Work out the finished part from the listing and answer in its coordinate system (mm). Give positions to 0.01 mm unless a question says otherwise; leave off trailing zeros. Loops run counter-clockwise (first coordinate to the right, second up) from the corner with the lowest first, then second, coordinate; pieces in that order, holes last. Notation, with made-up numbers: (89.25, -34.5) - (134.25, -34.5) arc R22 cw to (134.25, -11.5) - close; hole circle Ø6 at (67.25, 35). An arc over 180 degrees is marked (long way). One line per item, written item: value.
from build123d import *

# Parameters (mm, degrees)
SKETCH1_R           = 1.599999998
SKETCH1_R_2         = 1.45
BOSS_EXTRUDE1_DEPTH = 2


with BuildPart() as part:
    # Sketch1 → Boss-Extrude1 (new body)
    with BuildSketch(Plane.XZ):
        with BuildLine():
            Line((16.181421483, -3.177760966), (9.872858324, -4.530534353))
            ThreePointArc((9.872858324, -4.530534353), (9.325880949, -4.494155653), (8.88026758, -4.174880875))
            ThreePointArc((8.88026758, -4.174880875), (8.049335418, -3.798153126), (7.258365077, -4.252837604))
            ThreePointArc((7.258365077, -4.252837604), (6.336866412, -4.705264718), (5.502330147, -4.107435892))
            ThreePointArc((5.502330147, -4.107435892), (0, -0.499999997), (-5.502330147, -4.107435892))
            ThreePointArc((-5.502330147, -4.107435892), (-6.336866412, -4.705264718), (-7.258365077, -4.252837604))
            ThreePointArc((-7.258365077, -4.252837604), (-8.049335418, -3.798153126), (-8.88026758, -4.174880875))
            ThreePointArc((-8.88026758, -4.174880875), (-9.325880949, -4.494155653), (-9.872858324, -4.530534353))
            Line((-9.872858324, -4.530534353), (-16.181421483, -3.177760966))
            ThreePointArc((-16.181421483, -3.177760966), (-18.749999999, 0), (-16.181421483, 3.177760966))
            Line((-16.181421483, 3.177760966), (-7.150681086, 5.114262981))
            ThreePointArc((-7.150681086, 5.114262981), (-6.698238018, 5.106573021), (-6.295506482, 4.900245189))
            ThreePointArc((-6.295506482, 4.900245189), (-5.464959808, 4.681269053), (-4.770928095, 5.187310858))
            ThreePointArc((-4.770928095, 5.187310858), (-4.48101085, 5.518641983), (-4.076896383, 5.693352662))
            Line((-4.076896383, 5.693352662), (-1.17489874, 6.239775137))
            ThreePointArc((-1.17489874, 6.239775137), (0, 6.34942366), (1.17489874, 6.239775137))
            Line((1.17489874, 6.239775137), (4.076896383, 5.693352662))
            ThreePointArc((4.076896383, 5.693352662), (4.48101085, 5.518641983), (4.770928095, 5.187310858))
            ThreePointArc((4.770928095, 5.187310858), (5.464959808, 4.681269053), (6.295506482, 4.900245189))
            ThreePointArc((6.295506482, 4.900245189), (6.698238018, 5.106573021), (7.150681086, 5.114262981))
            Line((7.150681086, 5.114262981), (16.181421483, 3.177760966))
            ThreePointArc((16.181421483, 3.177760966), (18.749999999, 0), (16.181421483, -3.177760966))
        make_face()
        with Locations(Location((-15.5, 0, 0), (0, 0, 90))):
            Circle(SKETCH1_R, mode=Mode.SUBTRACT)
        with Locations(Location((15.5, 0, 0), (0, 0, 270))):
            Circle(SKETCH1_R, mode=Mode.SUBTRACT)
        with Locations(Location((7.931558887, -1.04420954, 0), (0, 0, 270))):
            Circle(SKETCH1_R_2, mode=Mode.SUBTRACT)
        with Locations(Location((-7.931558887, -1.04420954, 0), (0, 0, 90))):
            Circle(SKETCH1_R_2, mode=Mode.SUBTRACT)
    extrude(amount=-BOSS_EXTRUDE1_DEPTH)


solid = part.part
1. A flat-ended cylindrical pin translates along its axis: pin 1 Ø1 at (x, y) = (8, 0.5) entering from -Z (3 decimals). Find the tip coordinate at first contact, or state that the pin passes through.
Output:
pin 1: stops at z = -3.995
2. Section A-A (z = -1.25) is taken. Write down the section's boundary in (x, y).
Output:
outline: (-18.5, 0) - (-16.5, 0) - (-16.5, 2) - (-18.5, 2) - close; (-14.5, 0) - (-9.37, 0) - (-9.37, 2) - (-14.5, 2) - close; (-6.5, 0) - (-2.9, 0) - (-2.9, 2) - (-6.5, 2) - close; (2.9, 0) - (6.5, 0) - (6.5, 2) - (2.9, 2) - close; (9.37, 0) - (14.5, 0) - (14.5, 2) - (9.37, 2) - close; (16.5, 0) - (18.5, 0) - (18.5, 2) - (16.5, 2) - close
3. Find the intervals of material crossed by line 1 along X through (y, z) = (1.5, 0); line 2 along X through (y, z) = (0.45, -2); line 3 along X through (y, z) = (1.7, 1.25), in increasing order.
Output:
line 1: x = -18.75 to -17.1, -13.9 to -8.94, -6.93 to 6.93, 8.94 to 13.9, 17.1 to 18.75
line 2: x = -18.06 to -9.02, -6.84 to -3.97, 3.97 to 6.84, 9.02 to 18.06
line 3: x = -18.5 to -16.5, -14.5 to 14.5, 16.5 to 18.5
4. The mould has two halves that part along Z. Classify faces 1 (the cylindrical face through (17.086, 0.986, 0.208)), 2 (the cylindrical face through (0.1, 1, -0.5)), 3 (the flat face through (11.6, 0.99, 4.16)): released by +Z, released by -Z, zero draft, split by the parting line, or undercut.
Output:
face 1: undercut
face 2: released by -Z
face 3: released by +Z
5. Section B-B (x = 15.5) is taken. Write down the section's boundary in (y, z), and give its area (3 significant figures).
Output:
outline: (0, -3.32) - (2, -3.32) - (2, -1.6) - (0, -1.6) - close; (0, 1.6) - (2, 1.6) - (2, 3.32) - (0, 3.32) - close
area: 6.90 mm²
6. Section D-D (y = 1.2) is taken. Write down the section's boundary in (x, z).
Output:
outline: (-16.18, -3.18) - (-9.87, -4.53) arc R1 ccw to (-8.88, -4.17) arc R1 cw to (-7.26, -4.25) arc R1 ccw to (-5.5, -4.11) arc R6 cw to (5.5, -4.11) arc R1 ccw to (7.26, -4.25) arc R1 cw to (8.88, -4.17) arc R1 ccw to (9.87, -4.53) - (16.18, -3.18) arc R3.25 ccw to (16.18, 3.18) - (7.15, 5.11) arc R1 ccw to (6.3, 4.9) arc R1 cw to (4.77, 5.19) arc R1 ccw to (4.08, 5.69) - (1.17, 6.24) arc R6.35 ccw to (-1.17, 6.24) - (-4.08, 5.69) arc R1 ccw to (-4.77, 5.19) arc R1 cw to (-6.3, 4.9) arc R1 ccw to (-7.15, 5.11) - (-16.18, 3.18) arc R3.25 ccw to start; hole circle Ø3.2 at (-15.5, 0); hole circle Ø2.9 at (-7.93, -1.04); hole circle Ø2.9 at (7.93, -1.04); hole circle Ø3.2 at (15.5, 0)
7. Section C-C (z = 1) is taken. Write down the section's boundary in (x, y).
Output:
outline: (-18.59, 0) - (-16.75, 0) - (-16.75, 2) - (-18.59, 2) - close; (-14.25, 0) - (14.25, 0) - (14.25, 2) - (-14.25, 2) - close; (16.75, 0) - (18.59, 0) - (18.59, 2) - (16.75, 2) - close
